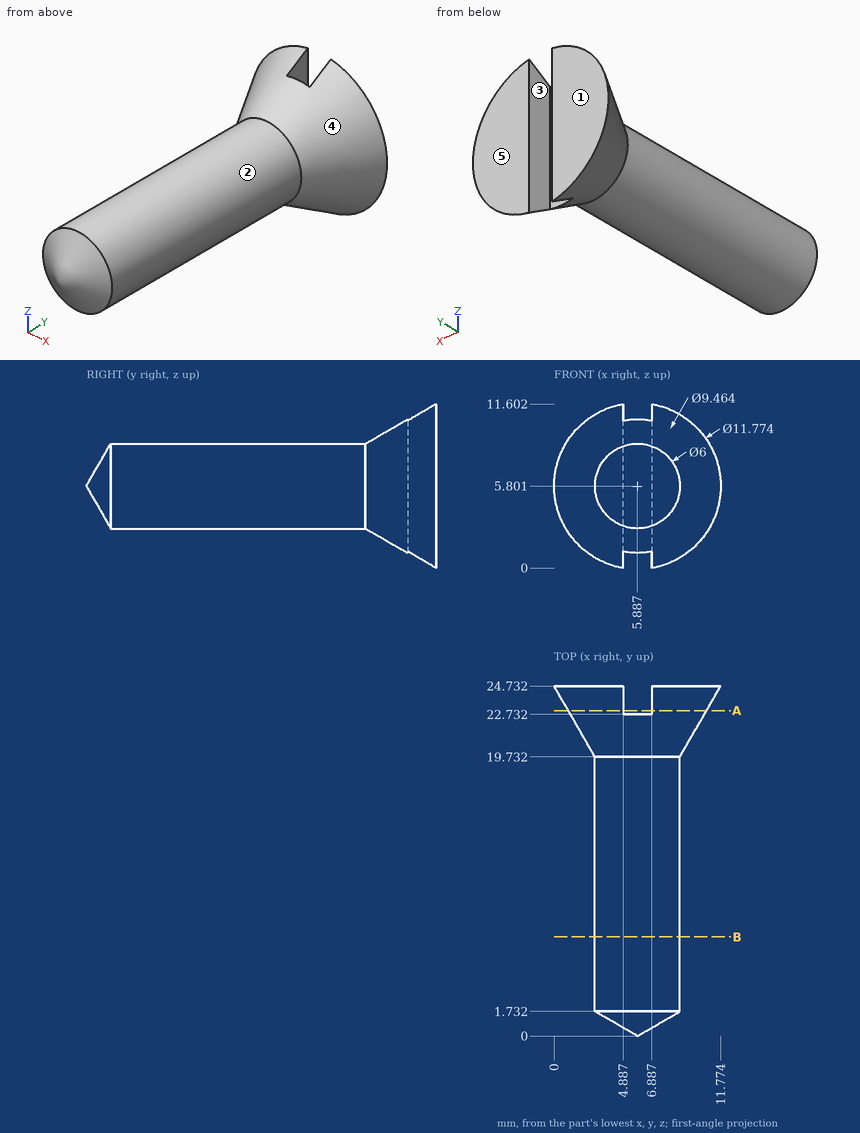
Answer from the drawing. Dimensions are ordinates in mm from the lowest x, y and z of the part. A direction names the side the tool comes from. Coordinates: 2 decimals unless noted, no trailing zeros. Write each loop counter-clockwise with the first axis right and the second up, starting at its lowest first coordinate (ties: lowest second). Pieces come first, ordered by that corner, then holes. Notation, with made-up numbers: (-33, 51.5) - (7, 51.5) arc R18 cw to (7, 75.5) - close; hole circle Ø11 at (27, 30.25). An arc over 180 degrees is marked (long way). Return JSON: item names as keys, results as strings.
1. For a pull along X with two mould halves and no side action, classify the marked faces 3, 4 and 5 as +X half, -X half, draft (parallel to the pull), parting line (faces both ways), or undercut.
Final values:
{"face 3": "undercut", "face 4": "parting line", "face 5": "draft"}
2. Each of these flat-tipped pins is pushed along its axis until it touches: pin 1 Ø6 at (x, y) = (4, 15) entering from -Z; pin 2 Ø1 at (y, z) = (23.5, 5) entering from +X; pin 3 Ø2 at (x, y) = (4.5, 20.5) entering from +Z. Where does it stop, or does it pass through?
Final values:
{"pin 1": "z = 2.8", "pin 2": "x = 11.3", "pin 3": "z = 9.65"}
3. The part is cut by section A-A on y = 23. Determine the outline of the cut face in (x, z) (1 decimal).
Final values:
{"outline": "(4.9, 1) - (4.9, 10.6) arc R4.9 ccw to start; (6.9, 1) arc R4.9 ccw to (6.9, 10.6) - close"}
4. Which of the six approach directions +Z, -Z, +X, -X, +Y, -Y give full straight-line access (tool end or side, diameter ignored) to the marked faces 1 and 2?
Final values:
{"face 1": "+Z, -Z, +X, -X, +Y", "face 2": "-Y"}
5. Consider line 1 along Z through (x, y) = (6, 10.5); line 2 along X through (y, z) = (12.5, 5.75); line 3 along Y through (x, z) = (7.75, 8.5) (1 decimal). Determine where each line is inside the solid, lowest interval first.
Final values:
{"line 1": "2.8 to 8.8", "line 2": "2.89 to 8.89", "line 3": "20.2 to 24.7"}
6. The part is cut by section B-B on y = 7. Determine the outline of the cut face in (x, z), then the cut area to 3 significant figures.
Final values:
{"outline": "circle Ø6 at (5.89, 5.8)", "area": "28.3 mm^2"}
